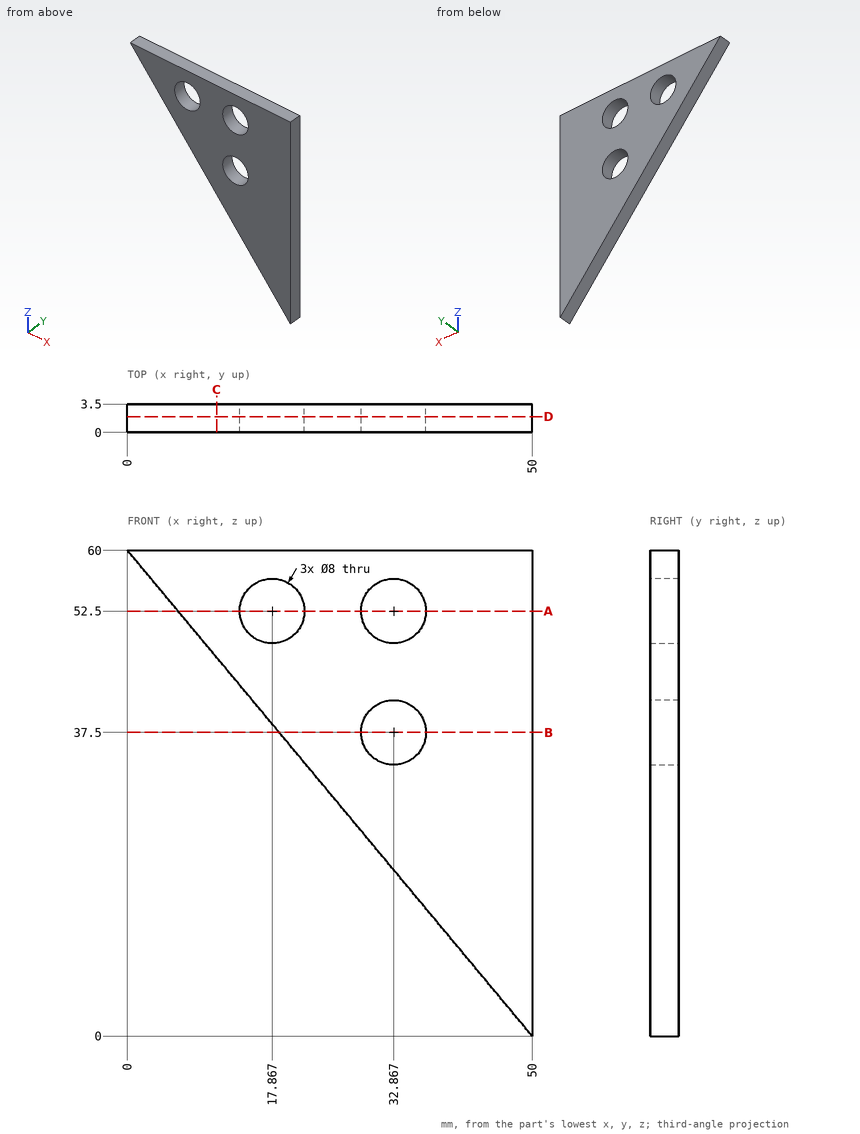
Part print with two shaded views. Sizes in mm from the minimum x, y, z corner. Coordinates: 2 decimals unless noted, no trailing zeros. Loops run counter-clockwise (first coordinate to the right, second up) from the corner with the lowest first, then second, coordinate; pieces in that order, holes last. Notation, with made-up numbers: (63, 7.5) -> (105, 7.5) arc R25 cw to (105, 40.5) -> close; hole circle Ø8 at (22.5, 1.25). An arc over 180 degrees is marked (long way). Answer as a JSON object with one key per item and string values.
Q1. Cut at A-A (z = 52.5). List the corners of the cut face in (x, y).
Report:
{"outline": "(6.25, 0) -> (13.87, 0) -> (13.87, 3.5) -> (6.25, 3.5) -> close; (21.87, 0) -> (28.87, 0) -> (28.87, 3.5) -> (21.87, 3.5) -> close; (36.87, 0) -> (50, 0) -> (50, 3.5) -> (36.87, 3.5) -> close"}
Q2. Cut at B-B (z = 37.5). List the corners of the cut face in (x, y).
Report:
{"outline": "(18.75, 0) -> (28.87, 0) -> (28.87, 3.5) -> (18.75, 3.5) -> close; (36.87, 0) -> (50, 0) -> (50, 3.5) -> (36.87, 3.5) -> close"}
Q3. Cut at D-D (y = 1.95). List the corners of the cut face in (x, z).
Report:
{"outline": "(0, 60) -> (50, 0) -> (50, 60) -> close; hole circle Ø8 at (17.87, 52.5); hole circle Ø8 at (32.87, 37.5); hole circle Ø8 at (32.87, 52.5)"}
Q4. Cut at C-C (x = 11). List the corners of the cut face in (y, z), and give its area (3 significant figures).
Report:
{"outline": "(0, 46.8) -> (3.5, 46.8) -> (3.5, 60) -> (0, 60) -> close", "area": "46.2 mm2"}
Q5. Probe probe 1 along X at (y, z) = (1.2, 52.5); probe 2 along X at (y, z) = (1.8, 39) (1 decimal); probe 3 along Z at (x, y) = (21, 2.85). List the from-to ranges inside material, lowest first.
Report:
{"probe 1": "x = 6.25 to 13.87, 21.87 to 28.87, 36.87 to 50", "probe 2": "x = 17.5 to 29.2, 36.6 to 50", "probe 3": "z = 34.8 to 50.01, 54.99 to 60"}
